Can you work these out from the drawing? Everything is in mm from the part's minimum corner. Coordinates: 2 decimals unless noted, no trailing zeros. Order: outer loops, then holes, each group sorted by start corner. A loop starts at its lowest first (then second) coordinate and runs counter-clockwise, first axis right, second up. Notation, with made-up numbers: (17, 33.5) -> (72, 33.5) arc R29 ccw to (72, 59.5) -> close; hole circle Ø4 at (63, -25.75). An arc over 180 degrees is marked (long way). Put each result on its own line as item: value. Start each with the question number.
Q1. If we section it at C-C (z = 217.5): Please give me the cut outline in (x, y).
Q2. We'd pull the mould along Z, two halves only. Please class the marked faces 1, 2 and 3: +Z half, -Z half, draft (parallel to the pull), parting line (faces both ways), or undercut.
Q3. If we section it at A-A (y = 5.5): Please give me the cut outline in (x, z).
Q4. Will these pins go through, and if not, where does the flat tip stop? pin 1 (12 mm diameter, centred on x = 187.5, y = 25.5, fed in from -Z); pin 2 (12 mm diameter, centred on x = 43, z = 155.5, fed in from -Y).
Q5. Please list where these lines run through material, in increasing order: line 1 along Z through (x, y) = (247, 5); line 2 along Y through (x, z) = (179, 57).
Q6. If we section it at B-B (x = 147.5): Please give me the cut outline in (y, z), and give its area (3 significant figures).
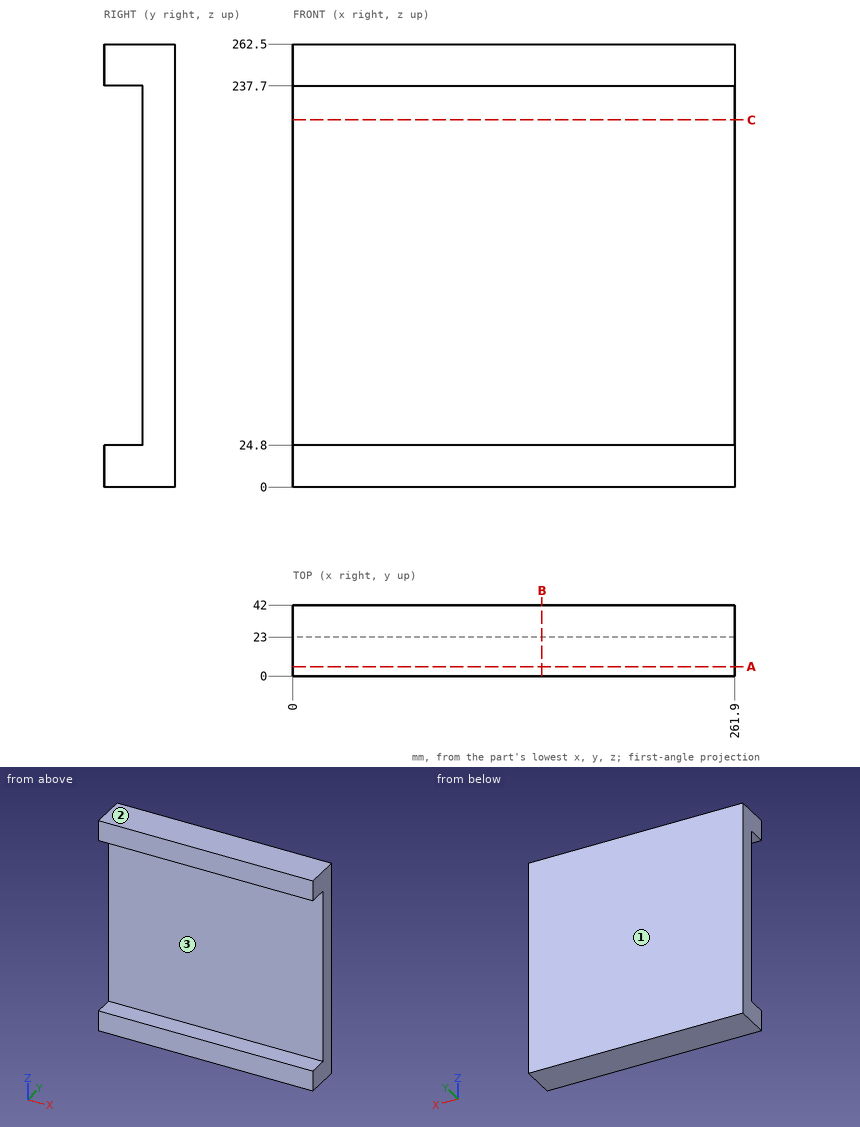
The answers:
1. outline: (0, 23) -> (261.9, 23) -> (261.9, 42) -> (0, 42) -> close
2. face 1: draft
2. face 2: +Z half
2. face 3: undercut
3. outline: (0, 0) -> (261.9, 0) -> (261.9, 24.8) -> (0, 24.8) -> close; (0, 237.7) -> (261.9, 237.7) -> (261.9, 262.5) -> (0, 262.5) -> close
4. pin 1: z = 0
4. pin 2: y = 23
5. line 1: 0 to 24.8, 237.7 to 262.5
5. line 2: 23 to 42
6. outline: (0, 0) -> (42, 0) -> (42, 262.5) -> (0, 262.5) -> (0, 237.7) -> (23, 237.7) -> (23, 24.8) -> (0, 24.8) -> close
6. area: 6,130 mm^2
